Autodesk Fusion 360 part; units mm, degrees
sketch "Sketch1" plane through (0, 0, 0) normal (0, 1, 0) x (1, 0, 0)
  line L0 (0, 0) -> (118.11, 0)
  line L1 (118.11, 0) -> (118.11, -187.325)
  line L2 (118.11, -187.325) -> (0, -187.325)
  line L3 (0, -187.325) -> (0, 0)
  dimension "d1" = 118.11
  dimension "d2" = 187.325
extrude "Extrude1" add sketch "Sketch1" along normal blind 11.43
fillet "Fillet1" radius 3.81 1 edges at (0, 5.715, 187.325)
sketch "Sketch2" plane through (118.11, 0, 0) normal (1, 0, 0) x (0, 1, 0)
  line L0 (0, 187.325) -> (0, 0)
  line L1 (0, 0) -> (11.43, 0)
  line L2 (11.43, 0) -> (11.43, 187.325)
  line L3 (11.43, 187.325) -> (0, 187.325)
  line L4 (5.08, 178.435) -> (8.255, 178.435)
  line L5 (8.255, 178.435) -> (8.255, 159.385)
  line L6 (8.255, 159.385) -> (5.08, 159.385)
  line L7 (5.08, 159.385) -> (5.08, 178.435)
  line L8 (5.08, 127.635) -> (8.255, 127.635)
  line L9 (8.255, 127.635) -> (8.255, 108.585)
  line L10 (8.255, 108.585) -> (5.08, 108.585)
  line L11 (5.08, 108.585) -> (5.08, 127.635)
  line L12 (5.08, 76.835) -> (8.255, 76.835)
  line L13 (8.255, 76.835) -> (8.255, 57.785)
  line L14 (8.255, 57.785) -> (5.08, 57.785)
  line L15 (5.08, 57.785) -> (5.08, 76.835)
  line L16 (5.08, 32.385) -> (8.255, 32.385)
  line L17 (8.255, 32.385) -> (8.255, 13.335)
  line L18 (8.255, 13.335) -> (5.08, 13.335)
  line L19 (5.08, 13.335) -> (5.08, 32.385)
  line L20 (11.43, 8.001) -> (0, 8.001)
  line L21 (0, 8.001) -> (0, 3.429)
  line L22 (0, 3.429) -> (11.43, 3.429)
  line L23 (11.43, 3.429) -> (11.43, 8.001)
  line L24 (5.334, 32.131) -> (8.001, 32.131)
  line L25 (8.001, 32.131) -> (8.001, 13.589)
  line L26 (8.001, 13.589) -> (5.334, 13.589)
  line L27 (5.334, 13.589) -> (5.334, 32.131)
  line L28 (8.001, 76.581) -> (8.001, 58.039)
  line L29 (8.001, 58.039) -> (5.334, 58.039)
  line L30 (5.334, 58.039) -> (5.334, 76.581)
  line L31 (5.334, 76.581) -> (8.001, 76.581)
  line L32 (8.001, 127.381) -> (8.001, 108.839)
  line L33 (8.001, 108.839) -> (5.334, 108.839)
  line L34 (5.334, 108.839) -> (5.334, 127.381)
  line L35 (5.334, 127.381) -> (8.001, 127.381)
  line L36 (8.001, 178.181) -> (8.001, 159.639)
  line L37 (8.001, 159.639) -> (5.334, 159.639)
  line L38 (5.334, 159.639) -> (5.334, 178.181)
  line L39 (5.334, 178.181) -> (8.001, 178.181)
  dimension "d7" = 8.89
  dimension "d8" = 3.175
  dimension "d9" = 5.08
  dimension "d10" = 19.05
  dimension "d11" = 19.05
  dimension "d12" = 5.08
  dimension "d13" = 31.75
  dimension "d14" = 3.175
  dimension "d15" = 19.05
  dimension "d16" = 5.08
  dimension "d17" = 31.75
  dimension "d18" = 3.175
  dimension "d19" = 3.175
  dimension "d20" = 19.05
  dimension "d21" = 25.4
  dimension "d22" = 5.08
  dimension "d44" = 4.572
  dimension "d45" = 11.43
  dimension "d46" = 0.254
  dimension "d47" = 0.254
  dimension "d48" = 0.254
  dimension "d49" = 0.254
  dimension "d50" = 3.429
extrude "Extrude2" add sketch "Sketch2" along normal blind 6.35 contours L0 L2 L20 L21 L22 L23 | L24 L25 L26 L27 | L28 L29 L30 L31 | L32 L33 L34 L35 | L36 L37 L38 L39
sketch "Sketch3" plane through (0, 0, 0) normal (0, 0, -1) x (1, 0, 0)
  line L0 (118.11, 0) -> (0, 0)
  line L1 (0, 0) -> (0, -11.43)
  line L2 (0, -11.43) -> (118.11, -11.43)
  line L3 (118.11, -11.43) -> (118.11, 0)
  line L4 (6.35, -5.08) -> (25.4, -5.08)
  line L5 (25.4, -5.08) -> (25.4, -8.255)
  line L6 (25.4, -8.255) -> (6.35, -8.255)
  line L7 (6.35, -8.255) -> (6.35, -5.08)
  dimension "d25" = 19.05
  dimension "d26" = 3.175
  dimension "d27" = 6.35
  dimension "d38" = 5.08
extrude "Extrude3" add sketch "Sketch3" along normal blind 3.175 contours L4 L5 L6 L7
sketch "Sketch4" plane through (0, 0, 0) normal (0, -1, 0) x (1, 0, 0)
  arc A0 (3.81, 187.325) -> (0, 183.515) centre (3.81, 183.515) ccw
  line L0 (0, 183.515) -> (0, 0)
  line L1 (0, 0) -> (118.11, 0)
  line L2 (118.11, 0) -> (118.11, 3.429)
  line L3 (118.11, 187.325) -> (3.81, 187.325)
  line L4 (118.11, 3.429) -> (124.46, 3.429)
  line L5 (124.46, 3.429) -> (124.46, 8.001)
  line L6 (124.46, 8.001) -> (118.11, 8.001)
  line L7 (118.11, 8.001) -> (118.11, 187.325)
  point P0 (8.89, 169.545)
  point P1 (8.89, 10.16)
  dimension "d31" = 17.78
  dimension "d32" = 8.89
  dimension "d41" = 10.16
  dimension "d42" = 8.89
hole "Hole1" at (8.89, 0, 169.545) at (8.89, 0, 10.16) direction (0, 1, 0) diameter 4 depth 15.24 tip angle 180 counterbore diameter 8.255 counterbore depth 2.54
extrude "Extrude4" cut 1 faces at (12.7, 7.1967, -3.175) along direction (0, 0, 1) blind 3.175
sketch "Sketch6" plane through (0, 11.43, 0) normal (0, 1, 0) x (-1, 0, 0)
  circle A0 centre (-8.89, 169.545) radius 2
  circle A1 centre (-8.89, 10.16) radius 2
  arc A2 (0, 183.515) -> (-3.81, 187.325) centre (-3.81, 183.515) ccw
  line L0 (-3.81, 187.325) -> (-118.11, 187.325)
  line L1 (-118.11, 187.325) -> (-118.11, 8.001)
  line L2 (-118.11, 8.001) -> (-124.46, 8.001)
  line L3 (-124.46, 8.001) -> (-124.46, 3.429)
  line L4 (-124.46, 3.429) -> (-118.11, 3.429)
  line L5 (-118.11, 3.429) -> (-118.11, 0)
  line L6 (-118.11, 0) -> (0, 0)
  line L7 (0, 0) -> (0, 183.515)
  line L8 (-86.36, 0) -> (-35.56, 0)
  line L9 (-35.56, 0) -> (-35.56, 50.8)
  line L10 (-35.56, 50.8) -> (-86.36, 50.8)
  line L11 (-86.36, 50.8) -> (-86.36, 0)
  point P0 (-60.96, 187.325)
  point P1 (-60.96, 50.8)
  dimension "d51" = 50.8
  dimension "d52" = 50.8
extrude "Extrude5" cut sketch "Sketch6" against normal blind 5.08 contours L6 L8 L9 L10 L11
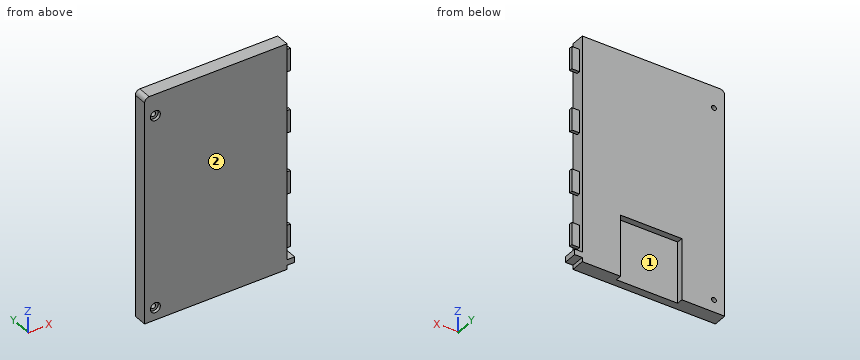
The listing builds one solid part. Answer for the finished solid, in the listing's coordinates (mm). Face numbers are marked on the shaded views. Give positions to 0.01 mm unless a question says otherwise; leave off trailing zeros. Order: outer loops, then holes, each group sorted by start corner. A loop starts at its lowest first (then second) coordinate and runs counter-clockwise, first axis right, second up. Notation, with made-up numbers: (36.25, 47) -> (68.25, 47) arc R9 cw to (68.25, 56) -> close; hole circle Ø4 at (-24.5, 32). An arc over 180 degrees is marked (long way). Answer as a JSON object with one key per item and string values. Group by question number.
Item 1: The part is cut by section B-B on x = 8.89. Write down the section's boundary in (y, z) (1 decimal), and give its area (3 significant figures).
Item 2: Flat-ended cylindrical pins translate along their axes: pin 1 (5.5 mm diameter, centred on y = 8.5, z = 33, fed in from -X); pin 2 (1.5 mm diameter, centred on x = 49.5, y = 9, fed in from -Z); pin 3 (2 mm diameter, centred on x = 120, y = 7.5, fed in from -Z); pin 4 (5 mm diameter, centred on x = 8.89, z = 10.16, fed in from -Y). Find the tip coordinate at first contact, or state that the pin passes through.
Item 3: The part is cut by section D-D on x = 49. Write down the section's boundary in (y, z) (3 decimals), and give its area (3 significant figures).
Item 4: The part is cut by section C-C on z = 42. Write down the section's boundary in (x, y).
Item 5: Consider L1, parallel to Z at x = 8.89, y = 5.5 (3 decimals); L2, parallel to Z at x = 8.89, y = 1.45 (1 decimal); L3, parallel to X at y = 10.25, z = 47.5. Determine where each line is inside the solid, lowest interval first. Write a range as from..to.
Item 6: The part is cut by section A-A on z = 10.16. Write down the section's boundary in (x, y), and give its area (3 significant figures).
Item 7: Determine the mould class of the marked faces 1 and 2 for opening direction X: pulls with the +X half, pulls with the -X half, needs draft (parallel to the pull), parting line crosses it, or undercut.
Result set:
{
 "1": {"outline": "(0, 0) -> (11.4, 0) -> (11.4, 8.2) -> (2.5, 8.2) -> (2.5, 6) -> (0, 6) -> close; (0, 14.3) -> (2.5, 14.3) -> (2.5, 12.2) -> (11.4, 12.2) -> (11.4, 167.5) -> (2.5, 167.5) -> (2.5, 165.4) -> (0, 165.4) -> close; (0, 173.7) -> (2.5, 173.7) -> (2.5, 171.5) -> (11.4, 171.5) -> (11.4, 187.3) -> (0, 187.3) -> close", "area": "2,030 mm²"},
 "2": {"pin 1": "x = 0", "pin 2": "z = 50.8", "pin 3": "z = 3.43", "pin 4": "y = 2.54"},
 "3": {"outline": "(0, 0) -> (6.35, 0) -> (6.35, 50.8) -> (11.43, 50.8) -> (11.43, 187.325) -> (0, 187.325) -> close", "area": "1,880 mm²"},
 "4": {"outline": "(0, 0) -> (118.11, 0) -> (118.11, 11.43) -> (86.36, 11.43) -> (86.36, 6.35) -> (35.56, 6.35) -> (35.56, 11.43) -> (0, 11.43) -> close"},
 "5": {"L1": "0..8.16, 12.16..167.545, 171.545..187.325", "L2": "0..6, 14.3..165.4, 173.7..187.3", "L3": "0..35.56, 86.36..118.11"},
 "6": {"outline": "(0, 0) -> (4.76, 0) -> (4.76, 2.54) -> (6.89, 2.54) -> (6.89, 11.43) -> (0, 11.43) -> close; (10.89, 2.54) -> (13.02, 2.54) -> (13.02, 0) -> (118.11, 0) -> (118.11, 11.43) -> (86.36, 11.43) -> (86.36, 6.35) -> (35.56, 6.35) -> (35.56, 11.43) -> (10.89, 11.43) -> close", "area": "1,040 mm²"},
 "7": {"face 1": "undercut", "face 2": "needs draft"}
}
